Autodesk Inventor part; units mm, degrees
ref_plane "YZ Plane" through (0, 0, 0) normal (1, 0, 0) x (0, 1, 0)
ref_plane "XZ Plane" through (0, 0, 0) normal (0, 1, 0) x (-1, 0, 0)
ref_plane "XY Plane" through (0, 0, 0) normal (0, 0, 1) x (1, 0, 0)
sketch "Sketch1" plane through (0, 0, 0) normal (0, 0, 1) x (1, 0, 0)
  line L0 (-29.75, -11.25) -> (29.75, -11.25)
  line L1 (29.75, -11.25) -> (29.75, 11.25)
  line L2 (29.75, 11.25) -> (-29.75, 11.25)
  line L3 (-29.75, 11.25) -> (-29.75, -11.25)
  line L4 (-29.75, -11.25) -> (29.75, 11.25) construction
  line L5 (29.75, -11.25) -> (-29.75, 11.25) construction
  point P0 (0, 0)
  dimension "d0" = 59.5
  dimension "d1" = 22.5
extrude "Extrusion1" add sketch "Sketch1" against normal blind 1.6
fillet "Fillet1" radius 1.5 4 edges at (29.75, 11.25, -0.8) (29.75, -11.25, -0.8) (-29.75, 11.25, -0.8) (-29.75, -11.25, -0.8)
sketch "Sketch2" plane through (0, 0, 0) normal (0, 0, 1) x (1, 0, 0)
  circle A0 centre (-14.379, 1.26) radius 4.75
  line L0 (-28.25, -11.25) -> (28.25, -11.25)
  line L1 (-29.75, 9.75) -> (-29.75, -9.75)
  point P0 (0, 0)
  dimension "d5" = 9.5
  dimension "d15" = 12.51
  dimension "d16" = 15.371
extrude "Extrusion2" cut sketch "Sketch2" against normal through all
sketch "Sketch3" plane through (0, 0, 0) normal (0, 0, 1) x (1, 0, 0)
  line L0 (-28.25, -11.25) -> (28.25, -11.25)
  circle A0 centre (5.985, 0.26) radius 3.25
  circle A1 centre (19.955, 0.26) radius 3.25
  point P0 (0, 0)
  dimension "d8" = 6.5
  dimension "d9" = 13.97
  dimension "d10" = 11.51
  dimension "d11" = 5.985
  dimension "d14" = 11.51
extrude "Extrusion3" cut sketch "Sketch3" against normal through all
sketch "Sketch4" plane through (0, 0, 0) normal (0, 0, 1) x (1, 0, 0)
  line L0 (-28.25, -11.25) -> (28.25, -11.25)
  line L1 (-29.75, 9.75) -> (-29.75, -9.75)
  circle A0 centre (-24.539, -0.14) radius 1.55
  point P0 (0, 0)
  point P1 (-28.349, -5.24)
  dimension "d17" = 6.01
  dimension "d18" = 1.401
  dimension "d19" = 3.1
  dimension "d20" = 3.81
  dimension "d21" = 5.1
extrude "Extrusion4" cut sketch "Sketch4" against normal through all
sketch "Sketch5" plane through (0, 0, 0) normal (0, 0, 1) x (1, 0, 0)
  line L0 (-29.75, 11.25) -> (29.75, 11.25) construction
  line L1 (29.75, 11.25) -> (29.75, -11.2473) construction
  line L2 (29.75, -11.2473) -> (-29.75, -11.2473) construction
  line L3 (-29.75, -11.2473) -> (-29.75, 11.25) construction
  line L4 (28.25, 11.25) -> (-28.25, 11.25)
  line L5 (-29.75, 9.75) -> (-29.75, -9.75)
  line L6 (29.75, -9.75) -> (29.75, 9.75)
  point P0 (0, 0)
decal "Decal1"
equation "\"d14\" = d10"
properties part number "frontPlate"
Build history of the part. All positions in model axes, mm. Give positions to 0.01 mm unless a question says otherwise; leave off trailing zeros. Write each loop counter-clockwise with the first axis right and the second up, starting at its lowest first coordinate (ties: lowest second). Pieces come first, ordered by that corner, then holes. Notation, with made-up numbers: (20.25, -37) - (46.25, -37) arc R19 cw to (46.25, -10) - close; hole circle Ø2 at (84.25, 3.25). An arc over 180 degrees is marked (long way). Use one line per item in the form item = value. Start each with the question number.
1. Probe line 1 (Y direction, x = 20, z = -0.05); line 2 (X direction, y = 1.5, z = -0.95); line 3 (Y direction, x = -17, z = -1.2). List the from-to ranges inside material, lowest first. Write a range as [from, to].
2. Band-saw the part on D-D on x = 18.5. Write the cut outline in (y, z).
3. Two-plate mould, pull along Y, no slides. Class faces 1 (the face through (0, 0, 0)), 2 (the face through (-29.32, 10.8, -0.81)), 3 (the face through (9.085, 1.236, -0.789)): released by +Y, released by -Y, zero draft, split by the parting line, or undercut.
4. Band-saw the part on A-A on x = 6. Write the cut outline in (y, z).
5. Band-saw the part on B-B on z = -0.6. Write the cut outline in (x, y) (3 decimals), plus the area to 3 significant figures.
6. Band-saw the part on C-C on y = 3. Write the cut outline in (x, z).
Conclusion:
q1.line_1 = [-11.25, -2.99], [3.51, 11.25]
q1.line_2 = [-29.75, -19.12], [-9.64, 2.98], [8.99, 16.95], [22.96, 29.75]
q1.line_3 = [-11.25, -2.7], [5.22, 11.25]
q2.outline = (-11.25, -1.6) - (-2.65, -1.6) - (-2.65, 0) - (-11.25, 0) - close; (3.17, -1.6) - (11.25, -1.6) - (11.25, 0) - (3.17, 0) - close
q3.face_1 = zero draft
q3.face_2 = released by +Y
q3.face_3 = undercut
q4.outline = (-11.25, -1.6) - (-2.99, -1.6) - (-2.99, 0) - (-11.25, 0) - close; (3.51, -1.6) - (11.25, -1.6) - (11.25, 0) - (3.51, 0) - close
q5.outline = (-29.75, -9.75) arc R1.5 ccw to (-28.25, -11.25) - (28.25, -11.25) arc R1.5 ccw to (29.75, -9.75) - (29.75, 9.75) arc R1.5 ccw to (28.25, 11.25) - (-28.25, 11.25) arc R1.5 ccw to (-29.75, 9.75) - close; hole circle Ø3.1 at (-24.539, -0.14); hole circle Ø9.5 at (-14.379, 1.26); hole circle Ø6.5 at (5.985, 0.26); hole circle Ø6.5 at (19.955, 0.26)
q5.area = 1,190 mm²
q6.outline = (-29.75, -1.6) - (-18.8, -1.6) - (-18.8, 0) - (-29.75, 0) - close; (-9.96, -1.6) - (4.24, -1.6) - (4.24, 0) - (-9.96, 0) - close; (7.73, -1.6) - (18.21, -1.6) - (18.21, 0) - (7.73, 0) - close; (21.7, -1.6) - (29.75, -1.6) - (29.75, 0) - (21.7, 0) - close
